The model under review builds one solid part; all positions refer to its coordinate system, in mm. A direction names the side the tool comes from. Give positions to 0.01 mm unless a question says otherwise; leave off trailing zeros. Loops run counter-clockwise (first coordinate to the right, second up) from the corner with the lowest first, then second, coordinate; pieces in that order, holes last. Notation, with made-up numbers: (65, 59) -> (99, 59) arc R38 cw to (99, 98) -> close; hole circle Ø4 at (-16, -22.75). An arc over 180 degrees is marked (long way). Write each question's results on one line, items separated by ' | '. Start each with the question number.
Q1. We need section B-B (z = -87.5). Write out the cut boundary in (x, y), plus the area to 3 significant figures.
Q2. Mouldability with a two-part tool opening along Z and no side actions: class faces 5 (the face through (-30, 7, 0)), 6 (the face through (-30, 1, -59)), 7 (the face through (-30, 6, -100)), 8 (the face through (-30.4, 15, -39.6)) as released by +Z, released by -Z, zero draft, split by the parting line, or undercut.
Q3. Wall thickness on L1, parallel to X at y = 11.25, z = -63; L2, parallel to X at y = 3.5, z = -16; L3, parallel to Z at x = -10.5, y = 12.25: over which ranges is each line inside the solid? List them lowest first. Write a range as [from, to].
Q4. Machinability: for faces 1 (the face through (-10, 8, -95)), 2 (the face through (-46.2, 4.85, -26.94)), 3 (the face through (-19.133, 4.095, -5.07)), 4 (the face through (-50, 8, -61)), which of the approach directions +Z, -Z, +X, -X, +Y, -Y give a long, thin tool a straight path to every point of the face, cutting with its end or side? Answer none if there is none.
Q5. Insertion check: pin 1 Ø5 at (x, y) = (-24, 8.09) entering from -Z; pin 2 Ø7 at (x, y) = (-34, 8.09) entering from -Z; pin 3 Ø3 at (y, z) = (7.5, -23) entering from -X. Each pin has a flat end and moves straight along its axis. Give the tip position at first contact, or say it passes through.
Q6. We need section C-C (z = -7.5). Write out the cut boundary in (x, y).
Q7. We need section A-A (x = -14). Write out the cut boundary in (y, z), plus the area to 3 significant figures.
Q8. We need section D-D (x = -34). Write out the cut boundary in (y, z).
from build123d import *

# Parameters (mm, degrees)
CROQUIS1_W              = 60
CROQUIS1_H              = 100
SALIENTE_EXTRUIR3_DEPTH = 15
CROQUIS2_W              = 40
CROQUIS2_H              = 80
CORTAR_EXTRUIR1_DEPTH   = 14
SALIENTE_EXTRUIR4_DEPTH = 14
CROQUIS4_R              = 4
CORTAR_EXTRUIR2_DEPTH   = 10
CROQUIS5_R              = 4
CORTAR_EXTRUIR3_DEPTH   = 11
CROQUIS7_R              = 5
CORTAR_EXTRUIR5_DEPTH   = 28


with BuildPart() as part:
    # Croquis1 → Saliente-Extruir3 (new body)
    with BuildSketch(Plane(origin=(0, 0, 0), x_dir=(1, 0, 0), z_dir=(0, 1, 0))):
        with Locations((-30, 50)):
            Rectangle(CROQUIS1_W, CROQUIS1_H)
    extrude(amount=SALIENTE_EXTRUIR3_DEPTH)

    # Croquis2 → Cortar-Extruir1 (cut)
    with BuildSketch(Plane(origin=(0, 15, 0), x_dir=(1, 0, 0), z_dir=(0, 1, 0))):
        with Locations((-30, 50)):
            Rectangle(CROQUIS2_W, CROQUIS2_H)
    extrude(amount=-CORTAR_EXTRUIR1_DEPTH, mode=Mode.SUBTRACT)

    # Croquis3 → Saliente-Extruir4 (add)
    with BuildSketch(Plane(origin=(0, 1, 0), x_dir=(1, 0, 0), z_dir=(0, 1, 0))):
        with BuildLine():
            Line((-50, 10), (-30, 10))
            Line((-30, 10), (-30, 40.028839229))
            ThreePointArc((-30, 40.028839229), (-40.702908507, 38.056709268), (-50, 32.399356809))
            Line((-50, 32.399356809), (-50, 10))
        make_face()
    extrude(amount=SALIENTE_EXTRUIR4_DEPTH)

    # Croquis4 → Cortar-Extruir2 (cut)
    with BuildSketch(Plane(origin=(0, 0, -100), x_dir=(-1, 0, 0), z_dir=(0, 0, -1))):
        with Locations((14, 8.093468363)):
            Circle(CROQUIS4_R)
        with Locations((24, 8.093468363)):
            Circle(CROQUIS4_R)
        with Locations((34, 8.093468363)):
            Circle(CROQUIS4_R)
        with Locations((44, 8.093468363)):
            Circle(CROQUIS4_R)
    extrude(amount=-CORTAR_EXTRUIR2_DEPTH, mode=Mode.SUBTRACT)

    # Croquis5 → Cortar-Extruir3 (cut)
    with BuildSketch(Plane(origin=(0, 0, -10), x_dir=(-1, 0, 0), z_dir=(0, 0, -1))):
        with Locations((20, 8)):
            Circle(CROQUIS5_R)
    extrude(amount=-CORTAR_EXTRUIR3_DEPTH, mode=Mode.SUBTRACT)

    # Croquis7 → Cortar-Extruir5 (cut)
    with BuildSketch(Plane.ZY.offset(60)):
        with Locations((-22.972155743, 7.895487944)):
            Circle(CROQUIS7_R)
    extrude(amount=-CORTAR_EXTRUIR5_DEPTH, mode=Mode.SUBTRACT)


solid = part.part
Output:
1) outline: (-60, 0) -> (0, 0) -> (0, 15) -> (-10, 15) -> (-10, 1) -> (-50, 1) -> (-50, 15) -> (-60, 15) -> close | area: 340 mm2
2) face 5: released by +Z | face 6: undercut | face 7: released by -Z | face 8: zero draft
3) L1: [-60, -50], [-10, 0] | L2: [-60, -30], [-10, 0] | L3: [-100, -90], [-10, 0]
4) face 1: -Z | face 2: -X | face 3: +Z | face 4: +Y
5) pin 1: z = -10 | pin 2: z = -40.02 | pin 3: x = -32
6) outline: (-60, 0) -> (0, 0) -> (0, 15) -> (-60, 15) -> close; hole circle Ø8 at (-20, 8)
7) outline: (0, -100) -> (4.09, -100) -> (4.09, -90) -> (1, -90) -> (1, -10) -> (15, -10) -> (15, 0) -> (0, 0) -> close; (12.09, -100) -> (15, -100) -> (15, -90) -> (12.09, -90) -> close | area: 300 mm2
8) outline: (0, -100) -> (4.09, -100) -> (4.09, -90) -> (1, -90) -> (1, -39.76) -> (15, -39.76) -> (15, 0) -> (0, 0) -> close; (12.09, -100) -> (15, -100) -> (15, -90) -> (12.09, -90) -> close; hole circle Ø10 at (7.9, -22.97)
